The figure shows three views and two pictorial views of one solid part (mm, origin at its lowest corner). Answer the questions. A direction names the side the tool comes from. Round coordinates to 2 decimals unless told otherwise and drop trailing zeros. Write each loop counter-clockwise with the first axis right and the second up, starting at its lowest first coordinate (ties: lowest second). Pieces come first, ordered by that corner, then holes. Notation, with made-up numbers: M 18.25,44.25 L 61.25,44.25 A16 cw 61.25,75.25 Z; hole C 9,38.25 d8. An arc over 180 degrees is marked long. One line per item, written item: value. Start each with the question number.
Q1. Find section A-A (z = 10.5). Write down the section's boundary in (x, y).
Q2. Given pin 1 Ø3 at (x, y) = (36, 3) entering from -Z; pin 2 Ø2 at (x, y) = (28.5, 6) entering from +Z; pin 3 Ø0.9 at (y, z) = (2, 8) entering from -X, each flat-ended and moving along its own axis, determine where each tip first touches the part or whether it passes through.
Q3. A tool of negligible diameter and unlimited length cuts with its end or side. For the marked faces 1, 2 and 3, from which of +Z, -Z, +X, -X, +Y, -Y can it reach the whole face along a straight path? Write none if from no direction.
Q4. Find section B-B (y = 5). Write down the section's boundary in (x, z).
Q5. Find section C-C (z = 21). Write down the section's boundary in (x, y).
Q6. Consider probe 1 along X at (y, z) = (5, 19); probe 2 along Z at (x, y) = (37.5, 7.25); probe 3 along Y at (x, z) = (42, 3.5). Determine where each line is inside the solid, lowest interval first.
Q7. Find section D-D (y = 2.25). Count the separate pieces of the cut face and the enclosed holes in it.
Q8. The mould has two halves that part along Z. Classify the marked faces 4, 5 and 6: released by +Z, released by -Z, zero draft, split by the parting line, or undercut.
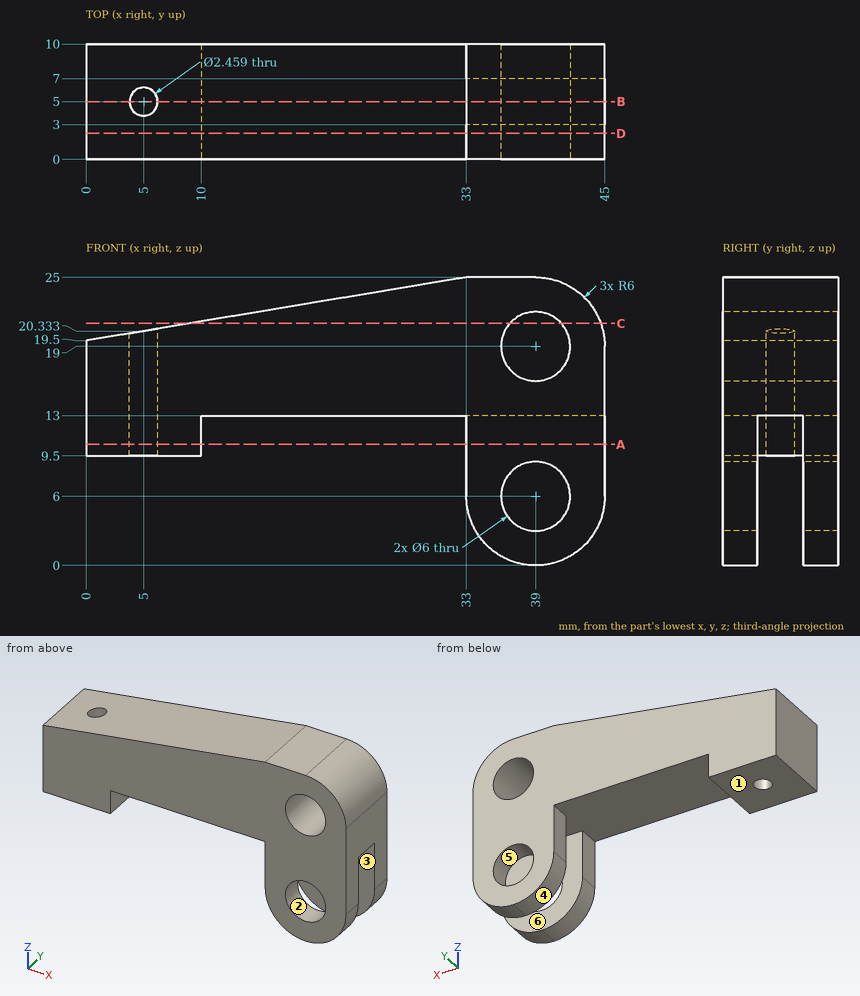
The answers:
1. outline: M 0,0 L 10,0 L 10,10 L 0,10 Z; M 33,0 L 45,0 L 45,3 L 33,3 Z; M 33,7 L 45,7 L 45,10 L 33,10 Z; hole C 5,5 d2.46
2. pin 1: z = 0.19
2. pin 2: z = 24.42
2. pin 3: x = 33
3. face 1: -Z, -X, +Y, -Y
3. face 2: +Y, -Y
3. face 3: -Z, +X
4. outline: M 0,9.5 L 3.77,9.5 L 3.77,20.13 L 0,19.5 Z; M 6.23,9.5 L 10,9.5 L 10,13 L 45,13 L 45,19 A6 ccw 39,25 L 33,25 L 6.23,20.54 Z; hole C 39,19 d6
5. outline: M 9,0 L 36.76,0 L 36.76,10 L 9,10 Z; M 41.24,0 L 44.66,0 L 44.66,10 L 41.24,10 Z
6. probe 1: 0 to 3.77, 6.23 to 36, 42 to 45
6. probe 2: 0.19 to 3.4, 8.6 to 16.4, 21.6 to 25
6. probe 3: 0 to 3, 7 to 10
7. separate pieces: 1
7. enclosed holes: 2
8. face 4: released by -Z
8. face 5: undercut
8. face 6: zero draft
